Geometry check sheet. Reference: the model listing, model coordinates, mm. A direction names the side the tool comes from. Coordinates: 2 decimals unless noted, no trailing zeros. Loops run counter-clockwise (first coordinate to the right, second up) from the corner with the lowest first, then second, coordinate; pieces in that order, holes last. Notation, with made-up numbers: (73.5, 13) - (131.5, 13) arc R21 ccw to (131.5, 50) - close; hole circle Ø3 at (-36, -39.75). An arc over 180 degrees is marked (long way). Write each question's results on one line, items separated by ' | '. Start each with the question number.
(1) Sectioned sample at A-A (z = -40). Enter the section's corners in (x, y).
(2) Sectioned sample at C-C (x = 35.5). Enter the section's corners in (y, z).
(3) Sectioned sample at B-B (y = -15). Enter the section's corners in (x, z).
(4) Mould release check, pull along Z, two halves, no side actions. Record for faces 1 (the face through (30, 0, -41)), 2 (the face through (12.1, -36.35, -68.3)), 3 (the face through (30, -15, 0)): pulls with the +Z half, pulls with the -Z half, needs draft (parallel to the pull), parting line crosses it, or undercut.
(5) Access from +Z, -Z, +X, -X, +Y, -Y to the whole of each face (thin tool, end or side, straight path). Record for faces 4 (the face through (51.8, -36.35, -15.5)), 5 (the face through (9.58, -38.23, -62.01)), 6 (the face through (46, -3.81, -39)).
(6) Material ranges on probe 1 along X at (y, z) = (-3.5, -26); probe 2 along Y at (x, z) = (12, -40); probe 3 along Y at (x, z) = (23, -73), recorded low to high.
(7) Go/stop test with flat-tipped pins: pin 1 Ø4 at (y, z) = (-15, -40) entering from +X; pin 2 Ø18 at (x, z) = (36, -36.5) entering from -Y; pin 3 Ø2.5 at (x, z) = (47, -57) entering from +Y. Record where each tip stops, or that it passes through.
(8) Sectioned sample at D-D (z = -24.5). Enter the section's corners in (x, y).
from build123d import *

# Parameters (mm, degrees)
SKETCH1_W               = 59.999999888
SKETCH1_H               = 80
BOSS_EXTRUDE1_DEPTH     = 30
CUT_EXTRUDE1_DEPTH      = 81
SKETCH3_R               = 4.445
BOSS_EXTRUDE2_DEPTH     = 3.81
SKETCH4_R               = 2.54
BOSS_EXTRUDE3_DEPTH     = 2.54
SKETCH5_R               = 4.445
BOSS_EXTRUDE4_DEPTH     = 3.81
F_1_4_20_TAPPED_HOLE1_D = 5.1054


with BuildPart() as part:
    # Sketch1 → Boss-Extrude1 (new body)
    with BuildSketch(Plane(origin=(0, 0, 0), x_dir=(1, 0, 0), z_dir=(0, 1, 0))):
        with Locations((29.999999944, 40)):
            Rectangle(SKETCH1_W, SKETCH1_H)
    extrude(amount=-BOSS_EXTRUDE1_DEPTH)

    # Sketch2 → Cut-Extrude1 (cut, through all)
    with BuildSketch(Plane.XY):
        with BuildLine():
            ThreePointArc((13.97, -3.81), (11.275923164, -2.694076836), (10.16, 0))
            Line((10.16, 0), (10.16, -3.81))
            Line((10.16, -3.81), (13.97, -3.81))
        make_face()
        with BuildLine():
            Line((17.78, 0), (10.16, 0))
            ThreePointArc((10.16, 0), (11.275923164, -2.694076836), (13.97, -3.81))
            ThreePointArc((13.97, -3.81), (16.664076836, -2.694076836), (17.78, 0))
        make_face()
        with BuildLine():
            ThreePointArc((17.78, 0), (16.664076836, -2.694076836), (13.97, -3.81))
            Line((13.97, -3.81), (17.78, -3.81))
            Line((17.78, -3.81), (17.78, 0))
        make_face()
        with BuildLine():
            Line((49.839999888, 0), (42.219999888, 0))
            ThreePointArc((42.219999888, 0), (43.335923052, -2.694076836), (46.029999888, -3.81))
            ThreePointArc((46.029999888, -3.81), (48.724076724, -2.694076836), (49.839999888, 0))
        make_face()
        with BuildLine():
            ThreePointArc((46.029999888, -3.81), (43.335923052, -2.694076836), (42.219999888, 0))
            Line((42.219999888, 0), (42.219999888, -3.81))
            Line((42.219999888, -3.81), (46.029999888, -3.81))
        make_face()
        with BuildLine():
            ThreePointArc((49.839999888, 0), (48.724076724, -2.694076836), (46.029999888, -3.81))
            Line((46.029999888, -3.81), (49.839999888, -3.81))
            Line((49.839999888, -3.81), (49.839999888, 0))
        make_face()
    extrude(amount=-CUT_EXTRUDE1_DEPTH, mode=Mode.SUBTRACT)

    # Sketch3 → Boss-Extrude2 (add)
    with BuildSketch(Plane.XZ.offset(30)):
        with Locations((49.839999888, -13.584)):
            Circle(SKETCH3_R)
        with Locations((10.16, -13.584)):
            Circle(SKETCH3_R)
        with Locations((49.839999888, -66.416)):
            Circle(SKETCH3_R)
        with Locations((10.16, -66.416)):
            Circle(SKETCH3_R)
    extrude(amount=BOSS_EXTRUDE2_DEPTH)

    # Sketch4 → Boss-Extrude3 (add)
    with BuildSketch(Plane.XZ.offset(33.81)):
        with Locations((49.839999888, -13.584)):
            Circle(SKETCH4_R)
        with Locations((10.16, -13.584)):
            Circle(SKETCH4_R)
        with Locations((10.16, -66.416)):
            Circle(SKETCH4_R)
        with Locations((49.839999888, -66.416)):
            Circle(SKETCH4_R)
    extrude(amount=BOSS_EXTRUDE3_DEPTH)

    # Sketch5 → Boss-Extrude4 (add)
    with BuildSketch(Plane.XZ.offset(36.35)):
        with Locations((10.16, -13.584)):
            Circle(SKETCH5_R)
        with Locations((10.16, -66.416)):
            Circle(SKETCH5_R)
        with Locations((49.839999888, -66.416)):
            Circle(SKETCH5_R)
        with Locations((49.839999888, -13.584)):
            Circle(SKETCH5_R)
    extrude(amount=BOSS_EXTRUDE4_DEPTH)

    # 1/4-20 Tapped Hole1 (through all)
    with Locations(Plane(origin=(59.999999888, 0, 0), x_dir=(0, 0, -1), z_dir=(1, 0, 0))):
        with Locations((40, -15)):
            Hole(F_1_4_20_TAPPED_HOLE1_D / 2)


solid = part.part
Outcome:
1) outline: (0, -30) - (60, -30) - (60, -17.55) - (0, -17.55) - close; (0, -12.45) - (60, -12.45) - (60, 0) - (49.84, 0) - (49.84, -3.81) - (42.22, -3.81) - (42.22, 0) - (17.78, 0) - (17.78, -3.81) - (10.16, -3.81) - (10.16, 0) - (0, 0) - close
2) outline: (-30, -80) - (0, -80) - (0, 0) - (-30, 0) - close; hole circle Ø5.11 at (-15, -40)
3) outline: (0, -80) - (60, -80) - (60, -42.55) - (0, -42.55) - close; (0, -37.45) - (60, -37.45) - (60, 0) - (0, 0) - close
4) face 1: needs draft | face 2: undercut | face 3: pulls with the +Z half
5) face 4: none | face 5: -Y | face 6: +Z, -Z, +Y
6) probe 1: x = 0 to 10.16, 17.78 to 42.22, 49.84 to 60 | probe 2: y = -30 to -17.55, -12.45 to -3.81 | probe 3: y = -30 to 0
7) pin 1: passes through | pin 2: stops at y = -30 | pin 3: stops at y = -3.81
8) outline: (0, -30) - (60, -30) - (60, 0) - (49.84, 0) - (49.84, -3.81) - (42.22, -3.81) - (42.22, 0) - (17.78, 0) - (17.78, -3.81) - (10.16, -3.81) - (10.16, 0) - (0, 0) - close
